Input: part model. Units: mm. Frame: model coordinates. A direction names the side the tool comes from. Give positions to 0.01 mm unless a question says otherwise; leave off trailing zeros. Order: outer loops, then holes, each group sorted by start corner. A loop starts at its lowest first (then second) coordinate and runs counter-clockwise, first axis right, second up. Notation, with made-up numbers: (68.25, 25) -> (107.25, 25) arc R20 ccw to (107.25, 29) -> close; hole circle Ø2 at (14.5, 87). An arc over 180 degrees is marked (long way). Use a Markdown table: item, result. Add a question column.
Autodesk Inventor part; units mm, degrees
ref_plane "YZ Plane" through (0, 0, 0) normal (1, 0, 0) x (0, 1, 0)
ref_plane "XZ Plane" through (0, 0, 0) normal (0, 1, 0) x (-1, 0, 0)
ref_plane "XY Plane" through (0, 0, 0) normal (0, 0, 1) x (1, 0, 0)
sketch "Sketch1" plane through (0, 0, 0) normal (0, 1, 0) x (-1, 0, 0)
  line L0 (9.5, 13) -> (-9.5, 13)
  line L1 (-9.5, 13) -> (-9.5, -13)
  line L2 (-9.5, -13) -> (9.5, -13)
  line L3 (9.5, -13) -> (9.5, 13)
  line L4 (9.5, 13) -> (-9.5, -13) construction
  line L5 (-9.5, 13) -> (9.5, -13) construction
  line L6 (7.5, 11) -> (-7.5, 11) construction
  line L7 (-7.5, 11) -> (-7.5, -11) construction
  line L8 (-7.5, -11) -> (7.5, -11) construction
  line L9 (7.5, -11) -> (7.5, 11) construction
  point P0 (0, 0)
  dimension "d0" = 19
  dimension "d1" = 26
  dimension "d2" = 2
extrude "Extrusion1" add sketch "Sketch1" against normal blind 1.5
sketch "Sketch2" plane through (0, 0, 0) normal (0, 1, 0) x (1, 0, 0)
  line L0 (-6, -19.9878) -> (6, -19.9878)
  line L1 (6, -19.9878) -> (6, -10.9878)
  line L2 (6, -10.9878) -> (-6, -10.9878)
  line L3 (-6, -10.9878) -> (-6, -19.9878)
  line L4 (-6, -19.9878) -> (6, -10.9878) construction
  line L5 (6, -19.9878) -> (-6, -10.9878) construction
  line L6 (-9.5, 13) -> (-9.5, -13)
  line L7 (-9.5, -13) -> (9.5, -13)
  point P0 (0, 0)
  point P1 (0, -15.4878)
  point P2 (0, -10.9878)
  point P3 (0, -10.9878)
  point P4 (0, -10.9878)
  dimension "d12" = 12
  dimension "d13" = 9
  dimension "d14" = 9.5
  dimension "d15" = 2.0122
extrude "Extrusion2" add sketch "Sketch2" along normal blind 4
sketch "Sketch3" plane through (0, 0, 0) normal (0, 1, 0) x (1, 0, 0)
  line L0 (-6, -6) -> (6, -6)
  line L1 (6, -6) -> (6, 6)
  line L2 (6, 6) -> (-6, 6)
  line L3 (-6, 6) -> (-6, -6)
  line L4 (-6, -6) -> (6, 6) construction
  line L5 (6, -6) -> (-6, 6) construction
  point P0 (0, 0)
  dimension "d18" = 12
  dimension "d19" = 12
hole "Hole2" at (-7.5, 0, 11) at (-7.5, 0, -11) direction (0, -1, 0) diameter 3 end through all
extrude "Extrusion3" add sketch "Sketch3" along normal blind 7
sketch "Sketch4" plane through (0, 7, 0) normal (0, 1, 0) x (1, 0, 0)
  circle A0 centre (0, 0) radius 3.25
  dimension "d29" = 6.5
extrude "Extrusion4" add sketch "Sketch4" along normal blind 4.5
sketch "Sketch5" plane through (0, 11.5, 0) normal (0, 1, 0) x (1, 0, 0)
  circle A0 centre (0, 0) radius 7
  dimension "d32" = 14
extrude "Extrusion5" add sketch "Sketch5" along normal blind 16.7
properties part number "encoder_footprint"
Q1. Ray query, line 1 (Z direction, x = -7.5, y = -1.2); line 2 (X direction, y = -0.7, z = 11); line 3 (Y direction, x = 0.25, z = 4). Return the intervals inside material, ascending.
Q2. Section query D-D (z = 0). Return loops of the section in (x, y), plus the area to 3 significant figures.
Q3. Section query C-C (x = 0). Return loops of the section in (y, z).
Q4. Draft query along Y for faces 1 (the cylindrical face through (-2.579, 9.218, -1.978)), 2 (the flat face through (0, 28.2, 0)), 3 (the flat face through (9.5, -1, 0)). Return one class per face: +Y half, -Y half, draft (parallel to the pull), parting line (faces both ways), or undercut.
Q5. Access query for faces 4 (the cylindrical face through (6.466, 19.733, -2.681)), 5 (the flat face through (0, 2, 10.988)), 6 (the flat face through (3, 11.5, -2)), 7 (the flat face through (0, 3, 6)), 8 (the flat face through (-6, 2, 15)). Directions: +Z, -Z, +X, -X, +Y, -Y. A direction counts if a zero-diameter tool reaches every point of the face in a straight line with its end or side. Return the directions, or none.
Q6. Section query A-A (z = -11). Return loops of the section in (x, y), plus the area to 3 significant figures.
Q7. First-contact query: pin 1 (2 mm diameter, centred on y = 1, z = 17.5, fed in from -X); pin 2 (4 mm diameter, centred on x = -7.5, z = -11, fed in from +Y); pin 3 (2 mm diameter, centred on x = 4, y = 4, fed in from -Z); pin 4 (5.5 mm diameter, centred on x = -4, z = 6.5, fed in from +Y). Flat tips, straight axial feed; report the tip coordinate or a pass-through.
Q8. Section query B-B (x = -7.5). Return loops of the section in (y, z).
Solution:
| question | item | result |
|---|---|---|
| 1 | line 1 | z = -13 to -12.5, -9.5 to 9.5, 12.5 to 13 |
| 1 | line 2 | x = -9.5 to -9, -6 to 9.5 |
| 1 | line 3 | y = -1.5 to 7, 11.5 to 28.2 |
| 2 | outline | (-9.5, -1.5) -> (9.5, -1.5) -> (9.5, 0) -> (6, 0) -> (6, 7) -> (3.25, 7) -> (3.25, 11.5) -> (7, 11.5) -> (7, 28.2) -> (-7, 28.2) -> (-7, 11.5) -> (-3.25, 11.5) -> (-3.25, 7) -> (-6, 7) -> (-6, 0) -> (-9.5, 0) -> close |
| 2 | area | 376 mm² |
| 3 | outline | (-1.5, -13) -> (0, -13) -> (0, -6) -> (7, -6) -> (7, -3.25) -> (11.5, -3.25) -> (11.5, -7) -> (28.2, -7) -> (28.2, 7) -> (11.5, 7) -> (11.5, 3.25) -> (7, 3.25) -> (7, 6) -> (0, 6) -> (0, 10.99) -> (4, 10.99) -> (4, 19.99) -> (0, 19.99) -> (0, 13) -> (-1.5, 13) -> close |
| 4 | face 1 | undercut |
| 4 | face 2 | +Y half |
| 4 | face 3 | draft |
| 5 | face 4 | +Y |
| 5 | face 5 | +X, -X, +Y |
| 5 | face 6 | none |
| 5 | face 7 | +X, -X |
| 5 | face 8 | +Z, -Z, -X, +Y |
| 6 | outline | (-9.5, -1.5) -> (-9, -1.5) -> (-9, 0) -> (-9.5, 0) -> close; (-6, -1.5) -> (9.5, -1.5) -> (9.5, 0) -> (-6, 0) -> close |
| 6 | area | 24.0 mm² |
| 7 | pin 1 | stops at x = -6 |
| 7 | pin 2 | stops at y = 0 |
| 7 | pin 3 | stops at z = -6 |
| 7 | pin 4 | stops at y = 28.2 |
| 8 | outline | (-1.5, -13) -> (0, -13) -> (0, -12.5) -> (-1.5, -12.5) -> close; (-1.5, -9.5) -> (0, -9.5) -> (0, 9.5) -> (-1.5, 9.5) -> close; (-1.5, 12.5) -> (0, 12.5) -> (0, 13) -> (-1.5, 13) -> close |
